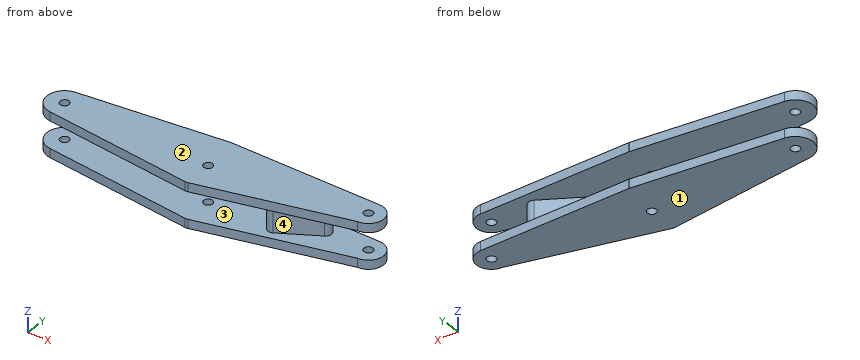
```python
from build123d import *

# Parameters (mm, degrees)
SKETCH1_R               = 3.81
BOSS_EXTRUDE1_DEPTH     = 38.1
CUT_EXTRUDE1_DEPTH      = 170.081733479
CUT_EXTRUDE1_DEPTH_BACK = 170.081733479
SKETCH2_W               = 296.702154824
SKETCH2_H               = 22.86
BOSS_EXTRUDE2_DEPTH     = 22.86
SCALE1_SCALE            = 2


with BuildPart() as part:
    # Sketch1 → Boss-Extrude1 (new body)
    with BuildSketch(Plane.XY):
        with BuildLine():
            Line((-147.344668758, 6.620564835), (-25.355087155, 20.167363089))
            ThreePointArc((-25.355087155, 20.167363089), (-24.906608979, 20.2037996), (-24.456762072, 20.213701798))
            Line((-24.456762072, 20.213701798), (102.089114394, 19.262041389))
            ThreePointArc((102.089114394, 19.262041389), (114.69360954, 6.562400496), (102.089114394, -6.137240398))
            Line((102.089114394, -6.137240398), (-19.792437318, -36.600949276))
            ThreePointArc((-19.792437318, -36.600949276), (-21.128759573, -36.811186783), (-22.481199669, -36.781813943))
            Line((-22.481199669, -36.781813943), (-147.344668758, -22.915873894))
            ThreePointArc((-147.344668758, -22.915873894), (-160.563675525, -8.14765453), (-147.344668758, 6.620564835))
        make_face()
        with Locations((-145.704675525, -8.14765453)):
            Circle(SKETCH1_R, mode=Mode.SUBTRACT)
        with Locations((101.99360954, 6.562400496)):
            Circle(SKETCH1_R, mode=Mode.SUBTRACT)
        with Locations((-21.120571626, -11.532910072)):
            Circle(SKETCH1_R, mode=Mode.SUBTRACT)
    extrude(amount=-BOSS_EXTRUDE1_DEPTH)

    # Sketch2 → Cut-Extrude1 (cut, two sides: drawn at the far end of the back side and taken through both)
    with BuildSketch(Plane(origin=(0, 0, 0), x_dir=(1, 0, 0), z_dir=(0, 1, 0)).offset(-CUT_EXTRUDE1_DEPTH_BACK)):
        with Locations((-25.145403948, 19.05)):
            Rectangle(SKETCH2_W, SKETCH2_H)
    extrude(amount=CUT_EXTRUDE1_DEPTH + CUT_EXTRUDE1_DEPTH_BACK, mode=Mode.SUBTRACT)


with BuildPart() as cut_extrude1_piece_1:
    # of the separate pieces the step leaves, piece 1, a body of its own (cut_extrude1_pieces)
    add(part.part.solids().sort_by_distance((-25.355087155, 20.167363089, -30.48))[0])



with BuildPart() as cut_extrude1_piece_2:
    # of the separate pieces the step leaves, piece 2, a body of its own (cut_extrude1_pieces)
    add(part.part.solids().sort_by_distance((-147.344668758, 6.620564835, 0))[0])


with BuildPart() as cut_extrude1_piece_1_1:
    add(cut_extrude1_piece_1.part)

    add(cut_extrude1_piece_2.part)  # Boss-Extrude2 merges Cut-Extrude1 piece 2
    # Sketch6 → Boss-Extrude2 (add)
    with BuildSketch(Plane.XY.offset(-30.48)):
        with BuildLine():
            Line((67.799114394, 2.317128757), (37.003251036, -15.462871243))
            ThreePointArc((37.003251036, -15.462871243), (30.063841985, -13.603462192), (31.923251036, -6.664053141))
            Line((31.923251036, -6.664053141), (62.719114394, 11.115946859))
            ThreePointArc((62.719114394, 11.115946859), (69.658523446, 9.256537808), (67.799114394, 2.317128757))
        make_face()
    extrude(amount=BOSS_EXTRUDE2_DEPTH)


with BuildPart() as cut_extrude1_piece_1_2:
    # Scale1: scaled about (-20.825252389, -4.795459228, -19.05)
    add(cut_extrude1_piece_1_1.part.scale(SCALE1_SCALE).moved(Location((20.825252389, 4.795459228, 19.05))))


solid = cut_extrude1_piece_1_2.part
```
Here's how the part is built. I have some questions about the finished solid (model axes, mm). Face numbers are marked on the shaded views. Give positions to 0.01 mm unless a question says otherwise; leave off trailing zeros. Loops run counter-clockwise (first coordinate to the right, second up) from the corner with the lowest first, then second, coordinate; pieces in that order, holes last. Notation, with made-up numbers: (37, 62.25) -> (48, 62.25) arc R26 cw to (48, 95.25) -> close; hole circle Ø11 at (40, -25.75). An arc over 180 degrees is marked (long way). Use one line per item in the form item = value. Start each with the question number.
1) Imagine slicing it at C-C (z = -48). Please give me the cut outline in (x, y).
2) Imagine slicing it at A-A (x = -160.5). Please give me the cut outline in (y, z), then the cut area to 3 significant figures.
3) Imagine slicing it at B-B (y = 35.5). Please give me the cut outline in (x, z).
4) Imagine slicing it at D-D (z = -12). Please give me the cut outline in (x, y).
5) For P1, Ø8, axis at y = 6.5, z = -21.5, coming from the -X side; P2, Ø1.5, axis at x = 88, z = -31.5, coming from the +Y side; P3, Ø4, axis at x = 141, z = -5, coming from the -Y side, each with a flat end and sliding along its axis, tell me the tip position at first contact or that it passes through.
6) Please list where these lines run through material, in increasing order: line 1 along Z through (x, y) = (-129, -41); line 2 along Y through (x, z) = (-63.5, -44); line 3 along Y through (x, z) = (-205, -42).
7) Thinking about a two-plate mould opening in Z: for the marked faces 1, 2, 3 and 4, which applies, +Z half, -Z half, draft (parallel to the pull), parting line (faces both ways), or undercut?
Check values:
q1.outline = (-273.86, -41.04) -> (-24.14, -68.77) arc R15.24 ccw to (-18.76, -68.41) -> (225, -7.48) arc R25.4 ccw to (225, 43.32) -> (-28.09, 45.22) arc R15.24 ccw to (-29.88, 45.13) -> (-273.86, 18.04) arc R29.72 ccw to start; hole circle Ø15.24 at (-270.58, -11.5); hole circle Ø15.24 at (-21.42, -18.27); hole circle Ø15.24 at (224.81, 17.92)
q2.outline = (-53.63, -57.15) -> (30.63, -57.15) -> (30.63, -41.91) -> (-53.63, -41.91) -> close; (-53.63, 3.81) -> (30.63, 3.81) -> (30.63, 19.05) -> (-53.63, 19.05) -> close
q2.area = 2,570 mm^2
q3.outline = (-116.61, -57.15) -> (243.15, -57.15) -> (243.15, -41.91) -> (-116.61, -41.91) -> close; (-116.61, 3.81) -> (243.15, 3.81) -> (243.15, 19.05) -> (-116.61, 19.05) -> close
q4.outline = (84.67, -8.53) arc R10.16 ccw to (94.83, -26.13) -> (156.42, 9.43) arc R10.16 ccw to (146.26, 27.03) -> close
q5.P1 = 103.78
q5.P2 = -6.18
q5.P3 = -0.63
q6.line_1 = -57.15 to -41.91, 3.81 to 19.05
q6.line_2 = -64.4 to 41.4
q6.line_3 = -48.68 to 25.68
q7.face_1 = -Z half
q7.face_2 = +Z half
q7.face_3 = undercut
q7.face_4 = undercut
